```python
from build123d import *

# Parameters (mm, degrees)
BOSS_EXTRUDE1_DEPTH                               = 24.13
SKETCH2_R                                         = 9.525
BOSS_EXTRUDE2_DEPTH                               = 15.25
CUT_EXTRUDE1_START                                = -15.25
SKETCH2_3_R                                       = 9.525
CUT_EXTRUDE1_DEPTH                                = 15.25
CUT_EXTRUDE1_DRAFT                                = -3
CBORE_FOR_5_16_SOCKET_HEAD_CAP_SCREW2_D           = 8.4328
CBORE_FOR_5_16_SOCKET_HEAD_CAP_SCREW2_CBORE_D     = 13.49502
CBORE_FOR_5_16_SOCKET_HEAD_CAP_SCREW2_CBORE_DEPTH = 7.9375
MIRROR1_START                                     = -15.25
MIRROR1_COPY_1_SKETCH_R                           = 9.525
MIRROR1_COPY_1_DEPTH                              = 15.25
MIRROR1_COPY_1_DRAFT                              = -3
FILLET1_R                                         = 2.54


with BuildPart() as part:
    # Sketch1 → Boss-Extrude1 (new body)
    with BuildSketch(Plane.XY):
        with BuildLine():
            Line((0, 50.8), (0, 38.1))
            ThreePointArc((0, 38.1), (38.1, 0), (0, -38.1))
            Line((0, -38.1), (0, -50.8))
            ThreePointArc((0, -50.8), (50.8, 0), (0, 50.8))
        make_face()
    extrude(amount=BOSS_EXTRUDE1_DEPTH)

    # Sketch2 → Boss-Extrude2 (add)
    with BuildSketch(Plane.ZY):
        with Locations((12.065, -50.8)):
            Circle(SKETCH2_R)
    boss_extrude2 = extrude(amount=-BOSS_EXTRUDE2_DEPTH)


with BuildPart() as cut_extrude1_tool:
    # Sketch2<3> → Cut-Extrude1 (with draft: the straight prism first)
    with BuildSketch(Plane.ZY.offset(CUT_EXTRUDE1_START)):
        with Locations((12.065, -50.8)):
            Circle(SKETCH2_3_R)
    extrude(amount=-CUT_EXTRUDE1_DEPTH)
    # Cut-Extrude1: the draft: its side faces are tilted about the plane it starts from
    cut_extrude1_sides = [cut_extrude1_tool.faces().sort_by_distance(p)[0] for p in [
        (22.875, -50.8, 2.54),
    ]]
    draft(cut_extrude1_sides, Plane.ZY.offset(CUT_EXTRUDE1_START), CUT_EXTRUDE1_DRAFT)


with BuildPart() as part_1:
    add(part.part)

    # Cut-Extrude1: cut by cut_extrude1_tool
    add(cut_extrude1_tool.part, mode=Mode.SUBTRACT)

    # CBORE for 5/16 Socket Head Cap Screw2 (through all)
    with Locations(Plane(origin=(15.25, -50.8, 12.065), x_dir=(0, 0, 1), z_dir=(1, 0, 0))):
        with Locations((0, 0)):
            cbore_for_5_16_socket_head_cap_screw2 = CounterBoreHole(CBORE_FOR_5_16_SOCKET_HEAD_CAP_SCREW2_D / 2, CBORE_FOR_5_16_SOCKET_HEAD_CAP_SCREW2_CBORE_D / 2, CBORE_FOR_5_16_SOCKET_HEAD_CAP_SCREW2_CBORE_DEPTH)

    # Mirror1: Boss-Extrude2, CBORE for 5/16 Socket Head Cap Screw2 across plane
    add(boss_extrude2.mirror(Plane.ZX))
    add(cbore_for_5_16_socket_head_cap_screw2.mirror(Plane.ZX), mode=Mode.SUBTRACT)


with BuildPart() as mirror1_copy_1_tool:
    # Mirror1 copy 1 sketch → Mirror1 copy 1 (with draft: the straight prism first)
    with BuildSketch(Plane.ZY.offset(MIRROR1_START)):
        with Locations((12.065, 50.8)):
            Circle(MIRROR1_COPY_1_SKETCH_R)
    extrude(amount=-MIRROR1_COPY_1_DEPTH)
    # Mirror1 copy 1: the draft: its side faces are tilted about the plane it starts from
    mirror1_copy_1_sides = [mirror1_copy_1_tool.faces().sort_by_distance(p)[0] for p in [
        (22.875, 50.8, 2.54),
    ]]
    draft(mirror1_copy_1_sides, Plane.ZY.offset(MIRROR1_START), MIRROR1_COPY_1_DRAFT)


with BuildPart() as part_2:
    add(part_1.part)

    # Mirror1 copy 1: cut by mirror1_copy_1_tool
    add(mirror1_copy_1_tool.part, mode=Mode.SUBTRACT)

    # Fillet1
    fillet1_edges = [part_2.edges().sort_by_distance(p)[0] for p in [
        (50.8, 0, 24.13),
        (50.8, 0, 0),
    ]]
    fillet(fillet1_edges, radius=FILLET1_R - 0.0001)  # a hair under: the kernel refuses the full size


solid = part_2.part
```
Check sheet for the modelled part. Datum: model origin and axes. Units: mm. A direction names the side the tool comes from. Round coordinates to 2 decimals unless told otherwise and drop trailing zeros. Write each loop counter-clockwise with the first axis right and the second up, starting at its lowest first coordinate (ties: lowest second). Pieces come first, ordered by that corner, then holes. Notation, with made-up numbers: M -34,14 L -12,14 A6 ccw -12,18 Z; hole C -21,-38.75 d4. An arc over 180 degrees is marked long. Write item = value, one per line. Start each with the question number.
1. Release check for a two-part mould opening along Y. For faces 3 (the conical face through (20.361, 41.544, 11.894)), 4 (the cylindrical face through (11.337, 44.213, 10.602)), 5 (the flat face through (0, 47, 15)) record: pulls with the +Y half, pulls with the -Y half, needs draft (parallel to the pull), parting line crosses it, or undercut.
2. Section check A-A, the plane y = 0. Record the cut outline in (x, z), then the cut area to 3 significant figures.
3. Scan lines: line 1 (Z direction, x = 5, y = 50.8); line 2 (Y direction, x = 14, z = 13.25); line 3 (Y direction, x = 10, z = 8). Record each from-to range of solid material in increasing order. Write a range as [from, to].
4. Tool access check on faces 1 (the flat face through (7.312, -50.9, 16.5)), 2 (the conical face through (20.353, -41.544, 12.236)). Record the directions out of +Z, -Z, +X, -X, +Y, -Y that give a thin tool (end or side, any length) a straight path to the whole face; none if there is none.
5. Gauge pin test, flat ends, axial feed: pin 1 (2 mm diameter, centred on x = 35, z = 13.5, fed in from +Y); pin 2 (10 mm diameter, centred on y = 36.5, z = 12, fed in from +X); pin 3 (12 mm diameter, centred on y = 36.5, z = 19, fed in from +X) (3 decimals). Record the tip position at first contact, or that the pin passes through.
6. Section check B-B, the plane x = 9. State how many separate pieces and enclosed holes the cut face has, then the cut area to 3 significant figures.
Results found:
q1.face_3 = pulls with the +Y half
q1.face_4 = undercut
q1.face_5 = needs draft
q2.outline = M 38.1,0 L 48.26,0 A2.54 ccw 50.8,2.54 L 50.8,21.59 A2.54 ccw 48.26,24.13 L 38.1,24.13 Z
q2.area = 304 mm^2
q3.line_1 = [2.54, 7.85], [16.28, 21.59]
q3.line_2 = [-60.25, -57.44], [-44.16, -35.43], [35.43, 44.16], [57.44, 60.25]
q3.line_3 = [-59.41, -56.19], [-45.41, -36.76], [36.76, 45.41], [56.19, 59.41]
q4.face_1 = +X
q4.face_2 = -Y
q5.pin_1 = 37.74
q5.pin_2 = 39.85
q5.pin_3 = 40.625
q6.separate_pieces = 2
q6.enclosed_holes = 2
q6.area = 650 mm^2
